Read the model definition and answer for the solid it produces. Units are mm, in the model's axes. Coordinates: 2 decimals unless noted, no trailing zeros. Loops run counter-clockwise (first coordinate to the right, second up) from the corner with the lowest first, then second, coordinate; pieces in that order, holes last. Notation, with made-up numbers: M -7,80 L 42,80 A28 ccw 42,101 Z; hole C -8.5,3.5 d5. An arc over 180 degrees is marked long. One line per item, written item: value. Start each with the question number.
```python
from build123d import *

# Parameters (mm, degrees)
SKETCH1_R           = 1.397
BOSS_EXTRUDE1_DEPTH = 0.4445
CUT_EXTRUDE4_DEPTH  = 16.51


with BuildPart() as part:
    # Sketch1 → Boss-Extrude1 (new body, symmetric)
    with BuildSketch(Plane.XY):
        with BuildLine():
            Line((9.00284972, 22.726912505), (9.71404972, 8.121912505))
            ThreePointArc((9.71404972, 8.121912505), (10.028030629, 7.257996655), (10.842675562, 6.832217089))
            ThreePointArc((10.842675562, 6.832217089), (11.725921803, -1.84754774), (13.772182249, -10.328777579))
            ThreePointArc((13.772182249, -10.328777579), (11.964609342, -11.463582415), (10.13976202, -10.356769839))
            Line((10.13976202, -10.356769839), (8.031181239, -2.228769839))
            ThreePointArc((8.031181239, -2.228769839), (7.732027762, -1.607745785), (7.219155962, -1.147174187))
            Line((7.219155962, -1.147174187), (6.050755962, -0.131174187))
            ThreePointArc((6.050755962, -0.131174187), (5.704248725, 0.270738994), (5.552221275, 0.779157252))
            Line((5.552221275, 0.779157252), (5.396674082, 1.769757252))
            ThreePointArc((5.396674082, 1.769757252), (5.343412822, 2.024518698), (5.192550751, 2.236605453))
            Line((5.192550751, 2.236605453), (4.709950751, 2.404757252))
            ThreePointArc((4.709950751, 2.404757252), (4.121509293, 2.682628498), (3.962230463, 3.313584941))
            Line((3.962230463, 3.313584941), (5.467671494, 15.403984941))
            ThreePointArc((5.467671494, 15.403984941), (6.633327736, 19.356034689), (9.00284972, 22.726912505))
        make_face()
        with Locations((7.503950751, 4.690757252)):
            Circle(SKETCH1_R, mode=Mode.SUBTRACT)
    extrude(amount=BOSS_EXTRUDE1_DEPTH, both=True)

    # Sketch2 → Cut-Extrude4 (cut)
    with BuildSketch(Plane(origin=(-1.247053398, 25.609132285, 0), x_dir=(0.998816471, 0.048638019, 0), z_dir=(-0.048638019, 0.998816471, 0))):
        Polygon((10.097586601, 0.4445), (10.097586601, -0.4445), (9.584322211, -0.4445), align=None)
    extrude(amount=-CUT_EXTRUDE4_DEPTH, mode=Mode.SUBTRACT)


solid = part.part
```
1) For a pull along X with two mould halves and no side action, classify faces 1 (the face through (6.643, -0.646, 0.006)), 2 (the face through (9, 2, 0.444)), 3 (the face through (6.47, 5.63, -0.01)), 4 (the face through (10.02, 7.27, 0.01)) as released by +X, released by -X, zero draft, split by the parting line, or undercut.
2) Section A-A (z = 0.05) is taken. Determine the outline of the cut face in (x, y).
3) Section C-C (y = 12) is taken. Determine the outline of the cut face in (x, z).
4) Section B-B (x = 13) is taken. Determine the outline of the cut face in (y, z), then the cut area to 3 significant figures.
5) Consider line 1 along Y through (x, z) = (7, 0.2); line 2 along Y through (x, z) = (7.5, -0.35); line 3 along X through (y, z) = (5, -0.1). Determine where each line is inside the solid, lowest interval first.
Results found:
1. face 1: released by -X
1. face 2: zero draft
1. face 3: undercut
1. face 4: released by +X
2. outline: M 3.96,3.31 A0.76 ccw 4.71,2.4 L 5.19,2.24 A0.64 cw 5.4,1.77 L 5.55,0.78 A1.27 ccw 6.05,-0.13 L 7.22,-1.15 A1.78 cw 8.03,-2.23 L 10.14,-10.36 A2.03 ccw 13.77,-10.33 A64.52 cw 10.84,6.83 A1.27 cw 9.71,8.12 L 9.64,9.61 L 9.36,9.6 L 8.73,22.44 A12.7 ccw 5.47,15.4 Z; hole C 7.5,4.69 d2.79
3. outline: M 5.04,-0.44 L 9.53,-0.44 L 9.01,0.44 L 5.04,0.44 Z
4. outline: M -11.17,-0.44 L -7.67,-0.44 L -7.67,0.44 L -11.17,0.44 Z
4. area: 3.11 mm²
5. line 1: y = -0.96 to 3.39, 5.99 to 20.06
5. line 2: y = -1.35 to 3.29, 6.09 to 20.87
5. line 3: x = 4.17 to 6.14, 8.87 to 10.93
